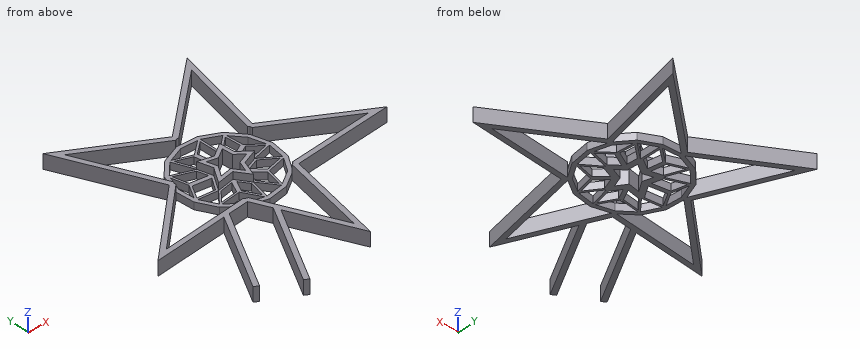
```python
from build123d import *

# Parameters (mm, degrees)
F1_DEPTH = 2.54
F2_DEPTH = 5.08
F3_DEPTH = 2.54


with BuildPart() as f1:
    # F0 (on Top) → F1 (new body)
    with BuildSketch(Plane.XY):
        Polygon((4.1629817264, 16.7427408623), (-2.2013881197, 16.9608854028), (-3.0068131679, 16.9884920758), (-3.5975513827, 16.7493756287), (-9.6567027493, 14.2967786738), (-14.636860697, 9.1330223569), (-16.819031361, 3.1255211535), (-17.0861724585, 2.3900835037), (-17.0408391317, 1.7477325928), (-16.5811297789, -4.7661225006), (-13.2090591257, -11.0982226257), (-8.1707658783, -15.0293453717), (-7.5530221491, -15.5113392346), (-6.9259689778, -15.6672522309), (-0.5909990259, -17.2424043737), (6.4732131979, -15.9921011543), (11.7815616344, -12.4065981462), (12.4181480525, -11.9766183616), (12.7489744416, -11.4464258818), (16.2158722935, -5.8902694501), (17.2097248984, 1.2145605608), (15.4482409163, 7.3426855737), (15.2278597229, 8.1093820168), (14.8271287482, 8.5863303821), (10.6129592606, 13.6020176507), align=None)
        Polygon((-8.87183017, 13.1347723613), (-8.2580116546, 13.3832311521), (-2.762426935, 15.6077100491), (3.1628166018, 15.4046169605), (3.8246250129, 15.3819328779), (4.0175995312, 15.2879667291), (9.6097206141, 12.5649643009), (9.7503645505, 12.4964797716), (10.3154122974, 11.8239622569), (13.990177478, 7.4502717858), (15.5683023366, 1.9600450691), (15.8109616228, 1.1158441247), (15.7892903314, 0.9609209091), (14.9276215775, -5.1989563128), (14.8978868649, -5.4115231227), (14.5693523604, -5.9380425585), (11.4088321251, -11.0031888601), (6.461372617, -14.3449308653), (5.9470866648, -14.6923032827), (5.7392984293, -14.7290799665), (-0.3884161265, -15.8136313636), (-0.5429641074, -15.8409849923), (-1.0821087258, -15.7069299285), (-6.9391314528, -14.250616486), (-11.6974519194, -10.5379421932), (-12.1354599299, -10.1961869264), (-12.2011743525, -10.0727878799), (-15.0780164622, -4.6706317106), (-15.233457138, -4.3787440178), (-15.300853021, -3.4237775529), (-15.6974512153, 2.1958235111), (-13.774064022, 7.4908955551), (-13.4472133706, 8.3907132065), (-13.3335565047, 8.5085601433), (-8.9854870359, 13.0169254245), align=None, mode=Mode.SUBTRACT)
    extrude(amount=F1_DEPTH)

    # F0 (on Top) → F2 (join)
    with BuildSketch(Plane.XY):
        Polygon((-33.6969470542, 35.9051802405), (-18.5940397475, 2.7332442428), (-44.1299353493, -20.8721632227), (-17.7662312147, -17.9002710145), (-15.6070743083, -17.6568764765), (-8.3429911406, -16.8380206717), (-5.2143965318, -23.5869952705), (-4.2844619667, -25.5930412891), (6.5595177125, -48.9855713404), (13.446561196, -13.1637173716), (48.2686344411, -9.6937073203), (16.6703053103, 8.6887283333), (24.1416345765, 42.6079515874), (-3.119114862, 18.5226071992), align=None)
        Polygon((-3.0068131679, 16.9884920758), (-2.2013881197, 16.9608854028), (21.2322100997, 37.6648753881), (14.8271287482, 8.5863303821), (15.2278597229, 8.1093820168), (15.4482409163, 7.3426855737), (42.6276437938, -8.4690246731), (12.7489744416, -11.4464258818), (12.4181480525, -11.9766183616), (11.7815616344, -12.4065981462), (5.8542420156, -43.2366020978), (-6.9259689778, -15.6672522309), (-7.5530221491, -15.5113392346), (-8.1707658783, -15.0293453717), (-38.9424450696, -18.498133868), (-17.0408391317, 1.7477325928), (-17.0861724585, 2.3900835037), (-16.819031361, 3.1255211535), (-29.8048108816, 31.6474102437), (-3.5975513827, 16.7493756287), align=None, mode=Mode.SUBTRACT)
        Polygon((-15.6070743083, -17.6568764765), (-17.7662312147, -17.9002710145), (-33.477195848, -46.6509044953), (-31.9222960033, -47.5132837729), align=None)
        Polygon((-4.2844619667, -25.5930412891), (-5.2143965318, -23.5869952705), (-21.4599514133, -53.315914213), (-19.9050526355, -54.1782928989), align=None)
    extrude(amount=F2_DEPTH)



with BuildPart() as f2:
    # F0 (on Top) → F2, piece 2 (new body)
    with BuildSketch(Plane.XY):
        Polygon((4.1200000644, 7.7903017796), (-0.7940794801, 4.4865484492), (-5.9754360801, 5.7629782777), (-4.5123451925, 0.6312052529), (-8.2113317605, -5.3255283132), (-1.9947032178, -4.096442149), (1.2593087084, -8.6874249228), (3.2795508064, -3.1629457339), (8.763532132, -0.9293583373), (4.5119235723, 2.4027612904), align=None)
        Polygon((-4.1539905478, 4.0062945987), (-0.5520264313, 3.1189489102), (3.0121522283, 5.5151590265), (3.2860576248, 1.749943662), (6.2573989827, -0.578790209), (2.2798709363, -2.1988096778), (0.897081895, -5.9801333565), (-1.4341748227, -2.6910367967), (-5.5907486439, -3.5128306902), (-3.1368822337, 0.4387998832), align=None, mode=Mode.SUBTRACT)
    extrude(amount=F2_DEPTH)


with BuildPart() as f1_1:
    add(f1.part)

    add(f2.part)  # F3 merges F2
    # F0 (on Top) → F3 (join)
    with BuildSketch(Plane.XY):
        Polygon((-4.5123451925, 0.6312052529), (-5.9754360801, 5.7629782777), (-13.3335565047, 8.5085601433), (-13.4472133706, 8.3907132065), (-13.774064022, 7.4908955551), (-12.3904388558, 1.7332251319), align=None)
        Polygon((-11.7914695166, 2.3932106743), (-13.0463627003, 7.6151895343), (-6.5817369362, 5.2030029646), (-5.5309745762, 1.5174671034), align=None, mode=Mode.SUBTRACT)
        Polygon((-8.2113317605, -5.3255283132), (-4.5123451925, 0.6312052529), (-12.3904388558, 1.7332251319), (-15.300853021, -3.4237775529), (-15.233457138, -4.3787440178), (-15.0780164622, -4.6706317106), align=None)
        Polygon((-14.7583322732, -3.961178532), (-11.9955596687, 0.9342160512), (-5.7350646244, 0.0584724657), (-8.5961228333, -4.5488871865), align=None, mode=Mode.SUBTRACT)
        Polygon((-0.7940794801, 4.4865484492), (-1.964637715, 11.1002015721), (-8.2580116546, 13.3832311521), (-8.87183017, 13.1347723613), (-8.9854870359, 13.0169254245), (-5.9754360801, 5.7629782777), align=None)
        Polygon((-5.4377678462, 6.3891455642), (-7.9717519008, 12.4958150767), (-2.6158103292, 10.5528552027), (-1.7166215483, 5.4724392849), align=None, mode=Mode.SUBTRACT)
        Polygon((3.1628166018, 15.4046169605), (-1.964637715, 11.1002015721), (-0.7940794801, 4.4865484492), (4.1200000644, 7.7903017796), (4.0175995312, 15.2879667291), (3.8246250129, 15.3819328779), align=None)
        Polygon((-0.2659681626, 5.7291925355), (-1.1651568481, 10.8096079145), (3.2910031409, 14.5504825172), (3.3780218404, 8.1790601046), align=None, mode=Mode.SUBTRACT)
        Polygon((9.6097206141, 12.5649643009), (4.1200000644, 7.7903017796), (4.5119235723, 2.4027612904), (10.8034854124, 5.7532438515), (10.3154122974, 11.8239622569), (9.7503645505, 12.4964797716), align=None)
        Polygon((4.8887121728, 7.3756327333), (4.881389673, 7.4762908036), (5.0001721085, 7.5796013524), (9.5962864589, 11.577053451), (10.0305084156, 6.1761429256), (5.1644805282, 3.5848083742), align=None, mode=Mode.SUBTRACT)
        Polygon((10.8034854124, 5.7532438515), (4.5119235723, 2.4027612904), (8.763532132, -0.9293583373), (15.7892903314, 0.9609209091), (15.8109616228, 1.1158441247), (15.5683023366, 1.9600450691), align=None)
        Polygon((5.8569437001, 2.2844957212), (10.7229715874, 4.8758302725), (14.9620662315, 1.5011510565), (8.9279294384, -0.1223325912), align=None, mode=Mode.SUBTRACT)
        Polygon((14.9276215775, -5.1989563128), (8.763532132, -0.9293583373), (3.2795508064, -3.1629457339), (7.9430756148, -7.6606580026), (14.5693523604, -5.9380425585), (14.8978868649, -5.4115231227), align=None)
        Polygon((8.1572798635, -6.8438879856), (4.6053955772, -3.418291642), (8.6719909478, -1.7619956724), (13.8661536119, -5.3597673452), align=None, mode=Mode.SUBTRACT)
        Polygon((7.9430756148, -7.6606580026), (3.2795508064, -3.1629457339), (1.2593087084, -8.6874249228), (5.7392984293, -14.7290799665), (5.9470866648, -14.6923032827), (6.461372617, -14.3449308653), align=None)
        Polygon((2.0874466636, -8.5675672358), (3.5827076434, -4.4786819617), (7.1345919298, -7.9042783053), (5.859837335, -13.654963535), align=None, mode=Mode.SUBTRACT)
        Polygon((1.2593087084, -8.6874249228), (-1.9947032178, -4.096442149), (-4.6486377456, -9.5467212497), (-1.0821087258, -15.7069299285), (-0.5429641074, -15.8409849923), (-0.3884161265, -15.8136313636), align=None)
        Polygon((-0.8661165856, -14.6098730783), (-3.8147970804, -9.5168296532), (-1.8767315973, -5.5367021526), (0.4671585391, -8.8436228043), align=None, mode=Mode.SUBTRACT)
        Polygon((-1.9947032178, -4.096442149), (-8.2113317605, -5.3255283132), (-12.2011743525, -10.0727878799), (-12.1354599299, -10.1961869264), (-11.6974519194, -10.5379421932), (-4.6486377456, -9.5467212497), align=None)
        Polygon((-11.1601935886, -9.8211437548), (-7.8689757469, -5.9051332795), (-3.1249878704, -4.9672020806), (-5.0716364955, -8.9649564363), align=None, mode=Mode.SUBTRACT)
    extrude(amount=F3_DEPTH)


solid = f1_1.part
```
Part model, mm, in its own coordinate system. Round coordinates to 2 decimals unless told otherwise and drop trailing zeros. Loops run counter-clockwise (first coordinate to the right, second up) from the corner with the lowest first, then second, coordinate; pieces in that order, holes last. Notation, with made-up numbers: (48, -40) -> (64, -40) arc R13 cw to (64, -36) -> close; hole circle Ø2 at (16, -6.5). An arc over 180 degrees is marked (long way). Use one line per item in the form item = value. Start each with the question number.
Item 1: Drop a flat-ended pin along its axis: pin 1 Ø3 at (x, z) = (-25, 3.5) entering from +Y. Give the stop position or say it passes through.
Item 2: Band-saw the part on A-A (z = 3.8). Give the number of separate pieces and of enclosed holes in the cut face, plus the area to 3 significant figures.
Item 3: Drill centre lines: line 1 along X through (y, z) = (-34.5, 1.9); line 2 along X through (y, z) = (25, 0.6); line 3 along Y through (x, z) = (-21.5, 2.05). Where is each one in solid material? Low to high.
Item 4: Band-saw the part on B-B (x = -26). List the corners of the cut face in (y, z), plus the area to 3 significant figures.
Data:
q1.pin_1 = 31.81
q2.separate_pieces = 2
q2.enclosed_holes = 2
q2.area = 776 mm^2
q3.line_1 = -26.84 to -24.81, -11.18 to -9.15, -0.16 to 1.8, 7.53 to 9.34
q3.line_2 = -28.73 to -26.78, -18.11 to -14.51, 4.21 to 6.9, 18.44 to 20.26
q3.line_3 = -28.44 to -24.73, -18.32 to -16.53, -2.37 to 0.05, 9.12 to 13.41, 26.93 to 28.97
q4.outline = (-36.68, 0) -> (-32.97, 0) -> (-32.97, 5.08) -> (-36.68, 5.08) -> close; (-18.83, 0) -> (-17.04, 0) -> (-17.04, 5.08) -> (-18.83, 5.08) -> close; (-6.53, 0) -> (-4.11, 0) -> (-4.11, 5.08) -> (-6.53, 5.08) -> close; (19, 0) -> (23.29, 0) -> (23.29, 5.08) -> (19, 5.08) -> close; (29.48, 0) -> (31.53, 0) -> (31.53, 5.08) -> (29.48, 5.08) -> close
q4.area = 72.4 mm^2
